Autodesk Inventor part; units mm, degrees
ref_plane "YZ Plane" through (0, 0, 0) normal (1, 0, 0) x (0, 1, 0)
ref_plane "XZ Plane" through (0, 0, 0) normal (0, 1, 0) x (-1, 0, 0)
ref_plane "XY Plane" through (0, 0, 0) normal (0, 0, 1) x (1, 0, 0)
sketch "Sketch1" plane through (0, 0, 0) normal (0, 0, 1) x (1, 0, 0)
  line L0 (-9, 30) -> (9, 30)
  line L1 (9, 30) -> (9, -30)
  line L2 (9, -30) -> (-9, -30)
  line L3 (-9, -30) -> (-9, 30)
  line L4 (-9, 30) -> (9, -30) construction
  line L5 (9, 30) -> (-9, -30) construction
  circle A0 centre (0, 0) radius 2.65
  circle A1 centre (0, 20) radius 2.65
  circle A2 centre (0, -20) radius 2.65
  dimension "d0" = 18
  dimension "d2" = 60
  dimension "d3" = 5.3
  dimension "d4" = 5.3
  dimension "d5" = 20
  dimension "d6" = 9
  dimension "d7" = 5.3
  dimension "d8" = 20
  dimension "d9" = 9
extrude "Extrusion1" add sketch "Sketch1" along normal blind 4
equation "\"d4\" = d3"
equation "\"d7\" = d3"
properties part number "3 Hole Joining Strip Plate" material "Aluminum 6061"
Geometry: final body of the model. Coordinates: model frame, mm. Give positions to 0.01 mm unless a question says otherwise; leave off trailing zeros. Loops run counter-clockwise (first coordinate to the right, second up) from the corner with the lowest first, then second, coordinate; pieces in that order, holes last. Notation, with made-up numbers: (16, -25) - (33, -25) arc R24 ccw to (33, 13) - close; hole circle Ø8 at (9, -3.5). An arc over 180 degrees is marked (long way). One line per question, with ' | ' between items. Start each with the question number.
(1) Pull-direction query (X, two-part tool) for faces 1 (the flat face through (-9, 0, 2)), 2 (the flat face through (0, -30, 2)), 3 (the cylindrical face through (1.425, -22.234, 1.972)); classes: released by +X, released by -X, zero draft, split by the parting line, or undercut.
(2) Section query A-A on y = 0. Return loops of the section in (x, z), then the cut area to 3 significant figures.
(3) Section query D-D on y = -21. Return loops of the section in (x, z), then the cut area to 3 significant figures.
(4) Section query C-C on z = 1.4. Return loops of the section in (x, y), then the cut area to 3 significant figures.
(5) Ray query, line 1 (Y direction, x = 0, z = 1.7); line 2 (X direction, y = -22, z = 3.55); line 3 (Y direction, x = 1.5, z = 1.75). Return the intervals inside material, ascending. Write a range as from..to.
(6) Section query B-B on x = 0. Return loops of the section in (y, z), then the cut area to 3 significant figures.
The answers:
1) face 1: released by -X | face 2: zero draft | face 3: undercut
2) outline: (-9, 0) - (-2.65, 0) - (-2.65, 4) - (-9, 4) - close; (2.65, 0) - (9, 0) - (9, 4) - (2.65, 4) - close | area: 50.8 mm2
3) outline: (-9, 0) - (-2.45, 0) - (-2.45, 4) - (-9, 4) - close; (2.45, 0) - (9, 0) - (9, 4) - (2.45, 4) - close | area: 52.4 mm2
4) outline: (-9, -30) - (9, -30) - (9, 30) - (-9, 30) - close; hole circle Ø5.3 at (0, -20); hole circle Ø5.3 at (0, 0); hole circle Ø5.3 at (0, 20) | area: 1,010 mm2
5) line 1: -30..-22.65, -17.35..-2.65, 2.65..17.35, 22.65..30 | line 2: -9..-1.74, 1.74..9 | line 3: -30..-22.18, -17.82..-2.18, 2.18..17.82, 22.18..30
6) outline: (-30, 0) - (-22.65, 0) - (-22.65, 4) - (-30, 4) - close; (-17.35, 0) - (-2.65, 0) - (-2.65, 4) - (-17.35, 4) - close; (2.65, 0) - (17.35, 0) - (17.35, 4) - (2.65, 4) - close; (22.65, 0) - (30, 0) - (30, 4) - (22.65, 4) - close | area: 176 mm2
